The model under review builds one solid part; all positions refer to its coordinate system, in mm. Give positions to 0.01 mm unless a question says otherwise; leave off trailing zeros. Write each loop counter-clockwise with the first axis right and the second up, starting at its lowest first coordinate (ties: lowest second). Pieces come first, ordered by that corner, then holes.
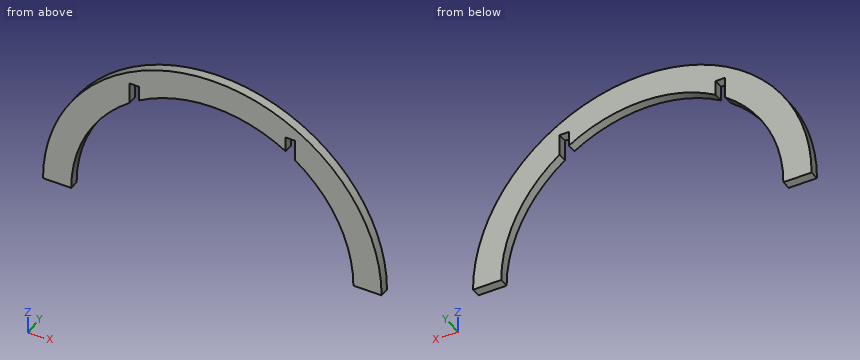
from build123d import *

# Parameters (mm, degrees)
F1_DEPTH = 6.35
F3_W     = 6.35
F3_H     = 6.35
F4_DEPTH = 30.48


with BuildPart() as f1:
    # F0 (on Front) → F1 (new body)
    with BuildSketch(Plane.XZ):
        with BuildLine():
            Line((95.25, 0), (114.3, 0))
            ThreePointArc((114.3, 0), (0, 114.3), (-114.3, 0))
            Line((-114.3, 0), (-95.25, 0))
            ThreePointArc((-95.25, 0), (0, 95.25), (95.25, 0))
        make_face()
    extrude(amount=F1_DEPTH)

    # F3 (on offset) → F4 (cut)
    with BuildSketch(Plane.XY.offset(60.96)):
        with Locations((-52.705, -3.175)):
            Rectangle(F3_W, F3_H)
        with Locations((52.705, -3.175)):
            Rectangle(F3_W, F3_H)
    extrude(amount=F4_DEPTH, mode=Mode.SUBTRACT)


solid = f1.part
1) Consider section A-A, the plane z = 26. Give the boundary of the cut face in (x, y).
2) Consider section D-D, the plane x = 0. Give the boundary of the cut face in (y, z).
3) Consider section C-C, the plane z = 13. Give the boundary of the cut face in (x, y).
4) Consider section B-B, the plane y = -5. Give the boundary of the cut face in (x, z), then the cut area to 3 significant figures.
5) To check wall thickness, follow probe 1 along X at (y, z) = (-3.25, 82); probe 2 along X at (y, z) = (-2.5, 33); probe 3 along X at (y, z) = (-4, 8). State the ranges of each line that lie inside material, in increasing order.
6) Insertion check: pin 1 (3 mm diameter, centred on y = -4, z = 87.5, fed in from -X); pin 2 (3 mm diameter, centred on x = 53, y = -3.5, fed in from -Z); pin 3 (1.5 mm diameter, centred on x = -82, y = -1.5, fed in from +Z). Each pin has a flat end and moves straight along its axis. Give the tip position at first contact, or say it passes through.
Answer block:
1. outline: (-111.3, -6.35) - (-91.63, -6.35) - (-91.63, 0) - (-111.3, 0) - close; (91.63, -6.35) - (111.3, -6.35) - (111.3, 0) - (91.63, 0) - close
2. outline: (-6.35, 95.25) - (0, 95.25) - (0, 114.3) - (-6.35, 114.3) - close
3. outline: (-113.56, -6.35) - (-94.36, -6.35) - (-94.36, 0) - (-113.56, 0) - close; (94.36, -6.35) - (113.56, -6.35) - (113.56, 0) - (94.36, 0) - close
4. outline: (-114.3, 0) - (-95.25, 0) arc R95.25 cw to (-55.88, 77.14) - (-55.88, 91.44) - (-49.53, 91.44) - (-49.53, 81.36) arc R95.25 cw to (49.53, 81.36) - (49.53, 91.44) - (55.88, 91.44) - (55.88, 77.14) arc R95.25 cw to (95.25, 0) - (114.3, 0) arc R114.3 ccw to start
4. area: 6,120 mm2
5. probe 1: x = -79.63 to -55.88, -49.53 to -48.46, 48.46 to 49.53, 55.88 to 79.63
5. probe 2: x = -109.43 to -89.35, 89.35 to 109.43
5. probe 3: x = -114.02 to -94.91, 94.91 to 114.02
6. pin 1: stops at x = -75.29
6. pin 2: stops at z = 91.44
6. pin 3: stops at z = 80.39
